Geometry: final body of the model. Coordinates: model frame, mm. Face numbers are marked on the shaded views. A direction names the side the tool comes from. Round coordinates to 2 decimals unless told otherwise and drop trailing zeros. Write each loop counter-clockwise with the first axis right and the second up, starting at its lowest first coordinate (ties: lowest second). Pieces come first, ordered by that corner, then holes.
from build123d import *

# Parameters (mm, degrees)
F0_W     = 30
F0_H     = 30
F1_DEPTH = 5
F3_DEPTH = 5
F4_W     = 5
F4_H     = 30
F5_DEPTH = 5


with BuildPart() as f1:
    # F0 (on Top) → F1 (new body)
    with BuildSketch(Plane.XY):
        with Locations((15, 15)):
            Rectangle(F0_W, F0_H)
    extrude(amount=F1_DEPTH)

    # F2 (on face) → F3 (join)
    with BuildSketch(Plane.XY.offset(5)):
        with BuildLine():
            Line((0, 30), (0, 19.584253))
            ThreePointArc((0, 19.584253), (15, 17.75), (30, 19.584253))
            Line((30, 19.584253), (30, 30))
            Line((30, 30), (0, 30))
        make_face()
        with BuildLine():
            Line((30, 0), (30, 13.93138))
            ThreePointArc((30, 13.93138), (15, 12.25), (0, 13.93138))
            Line((0, 13.93138), (0, 0))
            Line((0, 0), (30, 0))
        make_face()
    extrude(amount=F3_DEPTH)

    # F4 (on face) → F5 (join)
    with BuildSketch(Plane(origin=(0, 0, 0), x_dir=(1, 0, 0), z_dir=(0, 0, -1))):
        with Locations((8.5, -15)):
            Rectangle(F4_W, F4_H)
        with Locations((21.5, -15)):
            Rectangle(F4_W, F4_H)
    extrude(amount=F5_DEPTH)


solid = f1.part
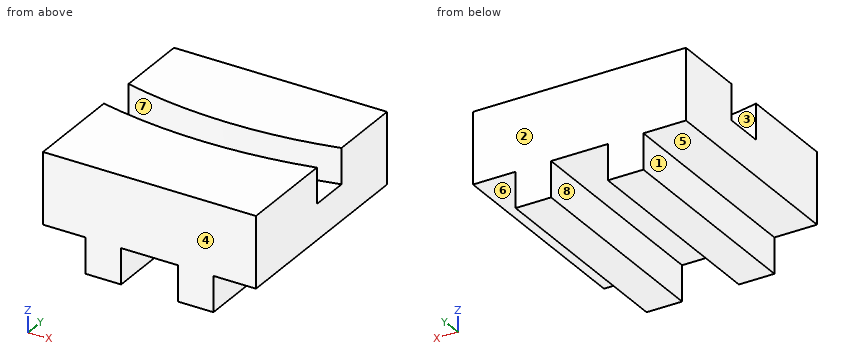
1) Section D-D on x = 28. Output: boundary loops of the cut face in (y, z), plus the area to 3 significant figures.
2) Section A-A on z = 8.25. Output: boundary loops of the cut face in (x, y).
3) Reachability of the marked faces 5, 6, 7 and 8 from +Z, -Z, +X, -X, +Y, -Y: full face, straight path, thin tool, end or side. Return the list, or none.
4) Line query: probe 1 along X at (y, z) = (15.75, -3.25); probe 2 along Z at (x, y) = (21.5, 18); probe 3 along Y at (x, z) = (17, 6.75). Output: solid intervals per line, ascending.
5) Section B-B on y = 21.75. Output: boundary loops of the cut face in (x, z), plus the area to 3 significant figures.
6) Section C-C on z = -1.25. Output: boundary loops of the cut face in (x, y), plus the area to 3 significant figures.
7) First-contact query: P1, Ø2.5, axis at y = 15, z = -1.5, coming from the +X side; P2, Ø4, axis at y = 15, z = -2.5, coming from the -X side; P3, Ø1.8, axis at x = 2.5, y = 14, coming from the -Z side. Flat tips, straight axial feed; report the tip coordinate or a pass-through.
8) Draft query along Y for the marked faces 1, 2, 3 and 4. Return one class per face: pulls with the +Y half, pulls with the -Y half, needs draft (parallel to the pull), parting line crosses it, or undercut.
Filled in:
1. outline: (0, 0) - (30, 0) - (30, 10) - (19.12, 10) - (19.12, 5) - (13.51, 5) - (13.51, 10) - (0, 10) - close
1. area: 272 mm2
2. outline: (0, 0) - (30, 0) - (30, 13.93) arc R67.75 cw to (0, 13.93) - close; (0, 19.58) arc R62.25 ccw to (30, 19.58) - (30, 30) - (0, 30) - close
3. face 5: -Z, -X, +Y, -Y
3. face 6: -Z, +X, +Y, -Y
3. face 7: +Z
3. face 8: -Z, +Y, -Y
4. probe 1: x = 6 to 11, 19 to 24
4. probe 2: z = -5 to 5
4. probe 3: y = 0 to 12.28, 17.78 to 30
5. outline: (0, 0) - (6, 0) - (6, -5) - (11, -5) - (11, 0) - (19, 0) - (19, -5) - (24, -5) - (24, 0) - (30, 0) - (30, 10) - (0, 10) - close
5. area: 350 mm2
6. outline: (6, 0) - (11, 0) - (11, 30) - (6, 30) - close; (19, 0) - (24, 0) - (24, 30) - (19, 30) - close
6. area: 300 mm2
7. P1: stops at x = 24
7. P2: stops at x = 6
7. P3: stops at z = 0
8. face 1: needs draft
8. face 2: pulls with the +Y half
8. face 3: undercut
8. face 4: pulls with the -Y half
